Design review of the part built by this model. Coordinates are the model's own, in mm. Face numbers are marked on the shaded views. A direction names the side the tool comes from. Give positions to 0.01 mm unless a question says otherwise; leave off trailing zeros. Order: outer loops, then holes, each group sorted by start corner. A loop starts at its lowest first (then second) coordinate and runs counter-clockwise, first axis right, second up. Notation, with made-up numbers: (71, 20.25) -> (107, 20.25) arc R29 cw to (107, 57.25) -> close; hole circle Ø10 at (29.25, 10). An arc over 180 degrees is marked (long way). Return JSON: item names as keys, results as strings.
Autodesk Inventor part; units mm, degrees
ref_plane "Work Plane1" through (0, 4, 0) normal (0, 1, 0) x (-1, 0, 0)
ref_plane "YZ Plane" through (0, 0, 0) normal (1, 0, 0) x (0, 1, 0)
ref_plane "XY Plane" through (0, 0, 0) normal (0, 0, 1) x (1, 0, 0)
sketch "Sketch1" plane through (0, 0, 0) normal (0, 1, 0) x (-1, 0, 0)
  line L0 (-4, 0) -> (-52, 0)
  line L1 (-56, -4) -> (-56, -47)
  line L2 (0, -47) -> (0, -4)
  line L3 (-19.75, -47) -> (-19.75, -55)
  line L4 (-19.75, -55) -> (-31.25, -55)
  line L5 (-31.25, -55) -> (-31.25, -47)
  line L6 (-7.75, -47) -> (-7.75, -43)
  line L7 (-7.75, -43) -> (-6.5, -43)
  line L8 (-6.5, -43) -> (-6.5, -40)
  line L9 (-6.5, -40) -> (-7.75, -40)
  line L10 (-7.75, -40) -> (-7.75, -35)
  line L11 (-7.75, -35) -> (-11.25, -35)
  line L12 (-11.25, -35) -> (-11.25, -40)
  line L13 (-11.25, -40) -> (-12.5, -40)
  line L14 (-12.5, -40) -> (-12.5, -43)
  line L15 (-12.5, -43) -> (-11.25, -43)
  line L16 (-11.25, -43) -> (-11.25, -47)
  line L17 (-36.25, -47) -> (-36.25, -43)
  line L18 (-36.25, -43) -> (-35, -43)
  line L19 (-35, -43) -> (-35, -40)
  line L20 (-35, -40) -> (-36.25, -40)
  line L21 (-36.25, -40) -> (-36.25, -35)
  line L22 (-36.25, -35) -> (-39.75, -35)
  line L23 (-39.75, -35) -> (-39.75, -40)
  line L24 (-39.75, -40) -> (-41, -40)
  line L25 (-41, -40) -> (-41, -43)
  line L26 (-41, -43) -> (-39.75, -43)
  line L27 (-39.75, -43) -> (-39.75, -47)
  line L28 (-19.75, -47) -> (-11.25, -47)
  line L29 (-7.75, -47) -> (0, -47)
  line L30 (-56, -47) -> (-39.75, -47)
  line L31 (-36.25, -47) -> (-31.25, -47)
  arc A0 (0, -4) -> (-4, 0) centre (-4, -4) ccw
  arc A1 (-52, 0) -> (-56, -4) centre (-52, -4) ccw
  point P0 (0, 0)
  point P1 (-56, 0)
  dimension "d0" = 56
  dimension "d1" = 47
  dimension "d2" = 8
  dimension "d3" = 11.5
  dimension "d4" = 19.75
  dimension "d5" = 4
  dimension "d6" = 3
  dimension "d7" = 5
  dimension "d8" = 3.5
  dimension "d9" = 6
  dimension "d10" = 7.75
  dimension "d11" = 3.5
  dimension "d12" = 6
  dimension "d13" = 16.25
  dimension "d14" = 4
extrude "Extrusion1" add sketch "Sketch1" along normal blind 8
sketch "Sketch2" plane through (0, 8, 0) normal (0, 1, 0) x (1, 0, 0)
  line L0 (56, 4) -> (56, 47) construction
  line L1 (56, 47) -> (39.75, 47) construction
  line L2 (39.75, 47) -> (39.75, 43) construction
  line L3 (39.75, 43) -> (41, 43) construction
  line L4 (41, 43) -> (41, 40) construction
  line L5 (41, 40) -> (39.75, 40) construction
  line L6 (39.75, 40) -> (39.75, 35) construction
  line L7 (39.75, 35) -> (36.25, 35) construction
  line L8 (36.25, 35) -> (36.25, 40) construction
  line L9 (36.25, 40) -> (35, 40) construction
  line L10 (35, 40) -> (35, 43) construction
  line L11 (35, 43) -> (36.25, 43) construction
  line L12 (36.25, 43) -> (36.25, 47) construction
  line L13 (36.25, 47) -> (31.25, 47) construction
  line L14 (31.25, 47) -> (31.25, 55) construction
  line L15 (31.25, 55) -> (19.75, 55) construction
  line L16 (19.75, 55) -> (19.75, 47) construction
  line L17 (19.75, 47) -> (11.25, 47) construction
  line L18 (11.25, 47) -> (11.25, 43) construction
  line L19 (11.25, 43) -> (12.5, 43) construction
  line L20 (12.5, 43) -> (12.5, 40) construction
  line L21 (12.5, 40) -> (11.25, 40) construction
  line L22 (11.25, 40) -> (11.25, 35) construction
  line L23 (11.25, 35) -> (7.75, 35) construction
  line L24 (7.75, 35) -> (7.75, 40) construction
  line L25 (7.75, 40) -> (6.5, 40) construction
  line L26 (6.5, 40) -> (6.5, 43) construction
  line L27 (6.5, 43) -> (7.75, 43) construction
  line L28 (7.75, 43) -> (7.75, 47) construction
  line L29 (7.75, 47) -> (0, 47) construction
  line L30 (0, 47) -> (0, 4) construction
  arc A0 (0, 4) -> (4, 0) centre (4, 4) ccw construction
  line L31 (4, 0) -> (52, 0) construction
  arc A1 (52, 0) -> (56, 4) centre (52, 4) ccw construction
  line L32 (21, 4) -> (52, 4) construction
  line L33 (52, 4) -> (52, 35) construction
  line L34 (52, 35) -> (21, 35) construction
  line L35 (21, 35) -> (21, 4) construction
  line L36 (21, 35) -> (52, 4) construction
  point P0 (0, 0)
  point P1 (36.5, 19.5)
  point P2 (10, 22.5)
  dimension "d17" = 31
  dimension "d18" = 31
  dimension "d19" = 4
  dimension "d20" = 4
  dimension "d21" = 22.5
  dimension "d22" = 10
hole "Hole1" at (21, 8, -35) at (52, 8, -35) at (52, 8, -4) at (21, 8, -4) direction (0, -1, 0) diameter 3.5 end through all
hole "Hole2" at (36.5, 8, -19.5) direction (0, -1, 0) diameter 23 end through all
hole "Hole3" at (10, 8, -22.5) direction (0, -1, 0) diameter 13 end through all
ref_plane "Work Plane1" through (0, 4, 0) normal (0, 1, 0) x (-1, 0, 0)
equation "\"d11\" = d8"
equation "\"d12\" = d9"
equation "\"d44\" = 0.5 * THICKNESS"
properties part number "A8-0003"
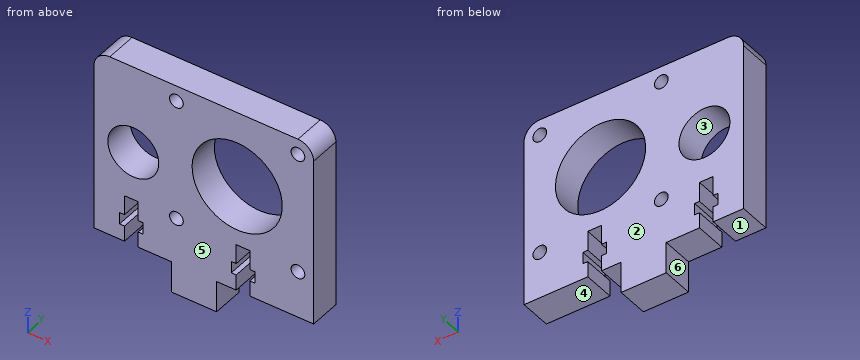
Item 1: Add section C-C (x = 10). Give the boundary of the cut face in (y, z).
Result set:
{"outline": "(0, -35) -> (8, -35) -> (8, -29) -> (0, -29) -> close; (0, -16) -> (8, -16) -> (8, 0) -> (0, 0) -> close"}
Item 2: Add section A-A (z = -44). Give the boundary of the cut face in (x, y).
Result set:
{"outline": "(0, 0) -> (7.75, 0) -> (7.75, 8) -> (0, 8) -> close; (11.25, 0) -> (36.25, 0) -> (36.25, 8) -> (11.25, 8) -> close; (39.75, 0) -> (56, 0) -> (56, 8) -> (39.75, 8) -> close"}
Item 3: Add section B-B (x = 21). Give the boundary of the cut face in (y, z).
Result set:
{"outline": "(0, -55) -> (8, -55) -> (8, -36.75) -> (0, -36.75) -> close; (0, -33.25) -> (8, -33.25) -> (8, -5.75) -> (0, -5.75) -> close; (0, -2.25) -> (8, -2.25) -> (8, 0) -> (0, 0) -> close"}
Item 4: Mouldability with a two-part tool opening along Z and no side actions: class the marked faces 1, 2 and 3 as released by +Z, released by -Z, zero draft, split by the parting line, or undercut.
Result set:
{"face 1": "released by -Z", "face 2": "zero draft", "face 3": "undercut"}
Item 5: Machinability: for the marked faces 4, 5 and 6, which of the approach directions +Z, -Z, +X, -X, +Y, -Y give a long, thin tool a straight path to every point of the face, cutting with its end or side? Answer none if there is none.
Result set:
{"face 4": "-Z, +X, +Y, -Y", "face 5": "+Z, -Z, +X, -X, -Y", "face 6": "-Z, -X, +Y, -Y"}
Item 6: Wall thickness on L1, parallel to X at y = 5.75, z = -37; L2, parallel to Z at x = 52, y = 4; L3, parallel to X at y = 6.25, z = -40.5: over which ranges is each line inside the solid? List them lowest first. Write a range as [from, to].
Result set:
{"L1": "x = [0, 7.75], [11.25, 36.25], [39.75, 56]", "L2": "z = [-47, -36.75], [-33.25, -5.75], [-2.25, 0]", "L3": "x = [0, 6.5], [12.5, 35], [41, 56]"}
Item 7: For pin 1 (2.5 mm diameter, centred on x = 50, y = 2.5, fed in from -Z), flat-tipped, find the tip position at first contact; note if it passes through.
Result set:
{"pin 1": "stops at z = -47"}
Item 8: Add section D-D (z = -12). Give the boundary of the cut face in (x, y).
Result set:
{"outline": "(0, 0) -> (27.78, 0) -> (27.78, 8) -> (0, 8) -> close; (45.22, 0) -> (56, 0) -> (56, 8) -> (45.22, 8) -> close"}
